```python
from build123d import *

# Parameters (mm, degrees)
SKETCH_1_W      = 30
SKETCH_1_H      = 30
EXTRUDE_1_DEPTH = 15
SKETCH_5_R      = 1.5
EXTRUDE_2_DEPTH = 2
FILLET_1_R      = 2


with BuildPart() as part:
    # Эскиз1 → Бобышка-Вытянуть1 (new body, symmetric)
    with BuildSketch(Plane(origin=(0, 0, 0), x_dir=(1, 0, 0), z_dir=(0, 1, 0))):
        Rectangle(SKETCH_1_W, SKETCH_1_H)
    extrude(amount=EXTRUDE_1_DEPTH, both=True)

    # Эскиз4 → Вырез-Повернуть1 (revolve, cut)
    with BuildSketch(Plane.XY):
        Polygon((-4.5, -15), (-4.5, -14), (-8.75, -9.75), (-8.75, 14), (-9.75, 15), (0, 15), (0, -15), align=None)
    cut_revolve_1 = revolve(axis=Axis((0, 15, 0), (0, -1, 0)), mode=Mode.SUBTRACT)

    # Эскиз5 → Бобышка-Вытянуть2 (add)
    with BuildSketch(Plane.XZ.offset(15)):
        with Locations(Location((-10, 7.5, 0), (0, 0, 270))):  # turned: the seam where the file's is
            Circle(SKETCH_5_R)
        with Locations(Location((-10, -7.5, 0), (0, 0, 270))):  # turned: the seam where the file's is
            Circle(SKETCH_5_R)
        with Locations(Location((10, -7.5, 0), (0, 0, 270))):  # turned: the seam where the file's is
            Circle(SKETCH_5_R)
        with Locations(Location((10, 7.5, 0), (0, 0, 270))):  # turned: the seam where the file's is
            Circle(SKETCH_5_R)
    extrude_2 = extrude(amount=EXTRUDE_2_DEPTH)

    # Зеркальное отражение1: Вырез-Повернуть1, Бобышка-Вытянуть2 across plane
    add(cut_revolve_1.mirror(Plane(origin=(0, 0, 0), x_dir=(0, 0, 1), z_dir=(0.707106781, 0.707106781, 0))), mode=Mode.SUBTRACT)
    add(extrude_2.mirror(Plane(origin=(0, 0, 0), x_dir=(0, 0, 1), z_dir=(0.707106781, 0.707106781, 0))))

    # Скругление1
    fillet_1_edges = [part.edges().sort_by_distance(p)[0] for p in [
        (-15, 15, 0),
        (0, 15, 15),
        (15, 15, 0),
        (0, -15, 15),
        (-15, -15, 0),
        (0, -15, -15),
        (15, 0, 15),
        (-15, 0, 15),
        (-15, 0, -15),
        (15, 0, -15),
        (0, 15, -15),
    ]]
    fillet(fillet_1_edges, radius=FILLET_1_R)


solid = part.part
```
Geometry: final body of the model. Coordinates: model frame, mm. A direction names the side the tool comes from. Round coordinates to 2 decimals unless told otherwise and drop trailing zeros. Write each loop counter-clockwise with the first axis right and the second up, starting at its lowest first coordinate (ties: lowest second). Pieces come first, ordered by that corner, then holes.
Item 1: Section query B-B (x = 12). Return loops of the section in (y, z), plus the area to 3 significant figures.
Item 2: Section query D-D (z = 11.75). Return loops of the section in (x, y).
Item 3: Pin query (flat end, axial travel): P1, Ø10.5, axis at y = 0, z = 0, coming from the +X side; P2, Ø1.5, axis at x = 10, z = -3, coming from the -Y side; P3, Ø14, axis at x = 0, z = 0, coming from the +Y side. Return the tip coordinate at first contact, or that it passes through.
Item 4: Set-up query: faces 4 (the face through (16, -10, -6)), 5 (the face through (1.2, -14.4, 14.43)), 6 (the face through (14.49, -0.59, -4.46)), 7 (the face through (6.45, -6.97, -5.91)), 8 (the face through (-10.9, -16, -6.3)). Return all of +Z, -Z, +X, -X, +Y, -Y with unobstructed straight access to the full face (end or side cutting, diameter ignored); none if empty.
Item 5: Mould query, pull axis X, two halves, no side actions, for faces 1 (the face through (9.1, -16, 8.7)), 2 (the face through (15, -4, 3)), 3 (the face through (16, 10.9, 8.7)). Classes: +X half, -X half, draft (parallel to the pull), parting line (faces both ways), or undercut.
Item 6: Section query A-A (y = 12). Return loops of the section in (x, z), plus the area to 3 significant figures.
Item 7: Material intervals for L1, parallel to Z at x = 0, y = -2; L2, parallel to Y at x = -5.5, z = 10; L3, parallel to Z at x = 11, y = 0, sorted ascending.
Item 8: Section query C-C (z = 0). Give the number of separate pieces and of enclosed holes in the cut face, plus the area to 3 significant figures.
Completed:
1. outline: (-15, -13) arc R2 ccw to (-13, -15) - (13, -15) arc R2 ccw to (15, -13) - (15, 13) arc R2 ccw to (13, 15) - (-13, 15) arc R2 ccw to (-15, 13) - close; hole circle Ø13 at (0, 0)
1. area: 764 mm2
2. outline: (-15, -13) arc R2 ccw to (-13, -15) - (15, -15) - (15, 13) arc R2 ccw to (13, 15) - (-13, 15) arc R2 ccw to (-15, 13) - close
3. P1: stops at x = 15
3. P2: stops at y = -15
3. P3: stops at y = -11.5
4. face 4: +X
4. face 5: +Z, +X, -X, -Y
4. face 6: +X, -X
4. face 7: +Y
4. face 8: -Y
5. face 1: undercut
5. face 2: +X half
5. face 3: draft
6. outline: (-15, -13) arc R2 ccw to (-13, -15) - (13, -15) arc R2 ccw to (15, -13) - (15, 13) arc R2 ccw to (13, 15) - (-13, 15) arc R2 ccw to (-15, 13) - close; hole circle Ø17.5 at (0, 0)
6. area: 656 mm2
7. L1: z = -15 to -8.75, 8.75 to 15
7. L2: y = -15 to 15
7. L3: z = -15 to -7.5, 7.5 to 15
8. separate pieces: 4
8. enclosed holes: 0
8. area: 205 mm2
